from build123d import *

# Parameters (mm, degrees)
BOSS_EXTRUDE1_DEPTH = 15
BOSS_EXTRUDE2_DEPTH = 15
BOSS_EXTRUDE4_DEPTH = 15
BOSS_EXTRUDE5_DEPTH = 15
SKETCH7_R           = 10
CUT_EXTRUDE1_DEPTH  = 15
SKETCH8_R           = 10
CUT_EXTRUDE2_DEPTH  = 15


with BuildPart() as part:
    # Sketch2 → Boss-Extrude1 (new body)
    with BuildSketch(Plane.XY):
        with BuildLine():
            Line((-60, 0), (60, 0))
            ThreePointArc((60, 0), (0, -60), (-60, 0))
        make_face()
    extrude(amount=BOSS_EXTRUDE1_DEPTH)

    # Sketch3 → Boss-Extrude2 (add)
    with BuildSketch(Plane.XY.offset(15)):
        with BuildLine():
            Line((-20, 30), (-20, 0))
            Line((-20, 0), (20, 0))
            Line((20, 0), (20, 30))
            ThreePointArc((20, 30), (0, 50), (-20, 30))
        make_face()
    extrude(amount=-BOSS_EXTRUDE2_DEPTH)

    # Sketch4 → Boss-Extrude4 (add)
    with BuildSketch(Plane.XY.offset(15)):
        with BuildLine():
            Line((20, 10), (20, 0))
            Line((20, 0), (29.123112456, 0.038520781))
            ThreePointArc((29.123112456, 0.038520781), (22.625419488, 3.246070605), (20, 10))
        make_face()
    extrude(amount=-BOSS_EXTRUDE4_DEPTH)

    # Sketch6 → Boss-Extrude5 (add)
    with BuildSketch(Plane.XY.offset(15)):
        with BuildLine():
            Line((-20, 10), (-20, 0))
            Line((-20, 0), (-30, 0))
            ThreePointArc((-30, 0), (-22.928932188, 2.928932188), (-20, 10))
        make_face()
    extrude(amount=-BOSS_EXTRUDE5_DEPTH)

    # Sketch7 → Cut-Extrude1 (cut)
    with BuildSketch(Plane.XY.offset(15)):
        with Locations((0, 30)):
            Circle(SKETCH7_R)
    extrude(amount=-CUT_EXTRUDE1_DEPTH, mode=Mode.SUBTRACT)

    # Sketch8 → Cut-Extrude2 (cut)
    with BuildSketch(Plane.XY.offset(15)):
        Circle(SKETCH8_R)
    extrude(amount=-CUT_EXTRUDE2_DEPTH, mode=Mode.SUBTRACT)


solid = part.part
Part model, mm, in its own coordinate system. A direction names the side the tool comes from. Coordinates: 2 decimals unless noted, no trailing zeros. Write each loop counter-clockwise with the first axis right and the second up, starting at its lowest first coordinate (ties: lowest second). Pieces come first, ordered by that corner, then holes. Notation, with made-up numbers: M 46.25,69 L 93.25,69 A17 ccw 93.25,82 Z; hole C 3,11 d3. An arc over 180 degrees is marked long. Return JSON: item names as keys, results as strings.
1. Pull direction Z, two halves, no side cores. Call faces 4 (the face through (1, -16, 0)), 5 (the face through (1, -16, 15)), 6 (the face through (1.319, -59.985, 7.395)): pulls with the +Z half, pulls with the -Z half, needs draft (parallel to the pull), parting line crosses it, or undercut.
Determined:
{"face 4": "pulls with the -Z half", "face 5": "pulls with the +Z half", "face 6": "needs draft"}
2. Saw through at D-D, the plane x = 27. Write the cut outline in (y, z).
Determined:
{"outline": "M -53.58,0 L 0,0 L 0,15 L -53.58,15 Z; M 0.03,0 L 0.46,0 L 0.46,15 L 0.03,15 Z"}
3. Flat gauge pins, fed straight in: pin 1 Ø8 at (y, z) = (-44.5, 9) entering from -X; pin 2 Ø10 at (x, y) = (4.5, -32.5) entering from -Z; pin 3 Ø3 at (y, z) = (-7, 2.5) entering from -X; pin 4 Ø7.5 at (x, z) = (42.5, 7.5) entering from +Y. Where does each tip first touch, or does it go through?
Determined:
{"pin 1": "x = -44.27", "pin 2": "z = 0", "pin 3": "x = -59.75", "pin 4": "y = 0"}
4. Saw through at B-B, the plane z = 7.5. Write the cut outline in (x, y).
Determined:
{"outline": "M -60,0 A60 ccw 60,0 L 20,0 L 29.12,0.04 A10 cw 20,10 L 20,30 A20 ccw -20,30 L -20,10 A10 cw -30,0 Z; hole C 0,0 d20; hole C 0,30 d20"}
5. Probe L1, parallel to Y at x = 0, z = 8.75; L2, parallel to Y at x = -3, z = 12; L3, parallel to X at y = 29, z = 12. List the from-to ranges inside material, lowest first.
Determined:
{"L1": "-60 to -10, 10 to 20, 40 to 50", "L2": "-59.92 to -9.54, 9.54 to 20.46, 39.54 to 49.77", "L3": "-20 to -9.95, 9.95 to 20"}
6. Saw through at C-C, the plane y = -4.5. Write the cut outline in (x, z), then the cut area to 3 significant figures.
Determined:
{"outline": "M -59.83,0 L -8.93,0 L -8.93,15 L -59.83,15 Z; M 8.93,0 L 59.83,0 L 59.83,15 L 8.93,15 Z", "area": "1,530 mm²"}
7. 3-axis set-ups, long thin cutter, end or side, ignore diameter. For faces 1 (the face through (0, 50, 8)), 2 (the face through (-20, 20, 8)), 3 (the face through (20, 20, 8)): which of +Z, -Z, +X, -X, +Y, -Y reach the whole face in a straight line?
Determined:
{"face 1": "+Z, -Z, +Y", "face 2": "+Z, -Z, -X, +Y", "face 3": "+Z, -Z, +X, +Y"}
8. Saw through at A-A, the plane x = 0. Write the cut outline in (y, z).
Determined:
{"outline": "M -60,0 L -10,0 L -10,15 L -60,15 Z; M 10,0 L 20,0 L 20,15 L 10,15 Z; M 40,0 L 50,0 L 50,15 L 40,15 Z"}
